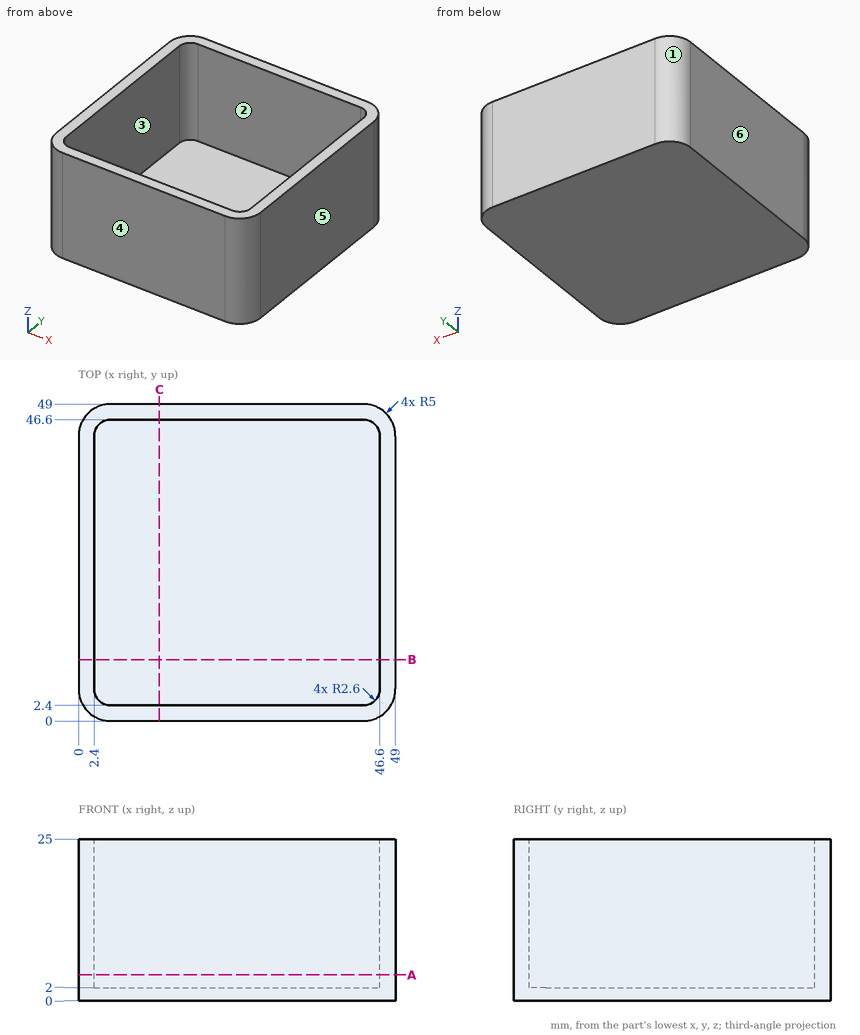
For this review, use the dimensioned drawing (mm, ordinates from the lowest corner) and the shaded views. A direction names the side the tool comes from. Coordinates: 2 decimals unless noted, no trailing zeros. Write each loop counter-clockwise with the first axis right and the second up, starting at its lowest first coordinate (ties: lowest second). Pieces come first, ordered by that corner, then holes. Notation, with made-up numbers: (27, 7.5) - (39, 7.5) arc R29 cw to (39, 32.5) - close; hole circle Ø5 at (-39.5, -6.5). An arc over 180 degrees is marked (long way). Answer as a JSON object with one key per item and string values. Group by question number.
1. To check wall thickness, follow probe 1 along X at (y, z) = (13, 20.5); probe 2 along Z at (x, y) = (20, 9.5). State the ranges of each line that lie inside material, in increasing order.
2. Add section B-B (y = 9.5). Give the boundary of the cut face in (x, z), plus the area to 3 significant figures.
3. Add section A-A (z = 4). Give the boundary of the cut face in (x, y), plus the area to 3 significant figures.
4. Mouldability with a two-part tool opening along X and no side actions: class the marked faces 3, 4, 5 and 6 as pulls with the +X half, pulls with the -X half, needs draft (parallel to the pull), parting line crosses it, or undercut.
5. Machinability: for the marked faces 1 and 2, which of the approach directions +Z, -Z, +X, -X, +Y, -Y give a long, thin tool a straight path to every point of the face, cutting with its end or side? Answer none if there is none.
6. Clearance check with a flat-ended pin moving along its axis: pin 1 Ø6 at (x, y) = (5.5, 24.5) entering from +Z. State where the tip first meets the part, or that it passes through.
Findings:
{
 "1": {"probe 1": "0 to 2.4, 46.6 to 49", "probe 2": "0 to 2"},
 "2": {"outline": "(0, 0) - (49, 0) - (49, 25) - (46.6, 25) - (46.6, 2) - (2.4, 2) - (2.4, 25) - (0, 25) - close", "area": "208 mm²"},
 "3": {"outline": "(0, 5) arc R5 ccw to (5, 0) - (44, 0) arc R5 ccw to (49, 5) - (49, 44) arc R5 ccw to (44, 49) - (5, 49) arc R5 ccw to (0, 44) - close; hole (2.4, 5) arc R2.6 ccw to (5, 2.4) - (44, 2.4) arc R2.6 ccw to (46.6, 5) - (46.6, 44) arc R2.6 ccw to (44, 46.6) - (5, 46.6) arc R2.6 ccw to (2.4, 44) - close", "area": "432 mm²"},
 "4": {"face 3": "undercut", "face 4": "needs draft", "face 5": "pulls with the +X half", "face 6": "pulls with the -X half"},
 "5": {"face 1": "+Z, -Z, -X, +Y", "face 2": "+Z"},
 "6": {"pin 1": "z = 2"}
}
